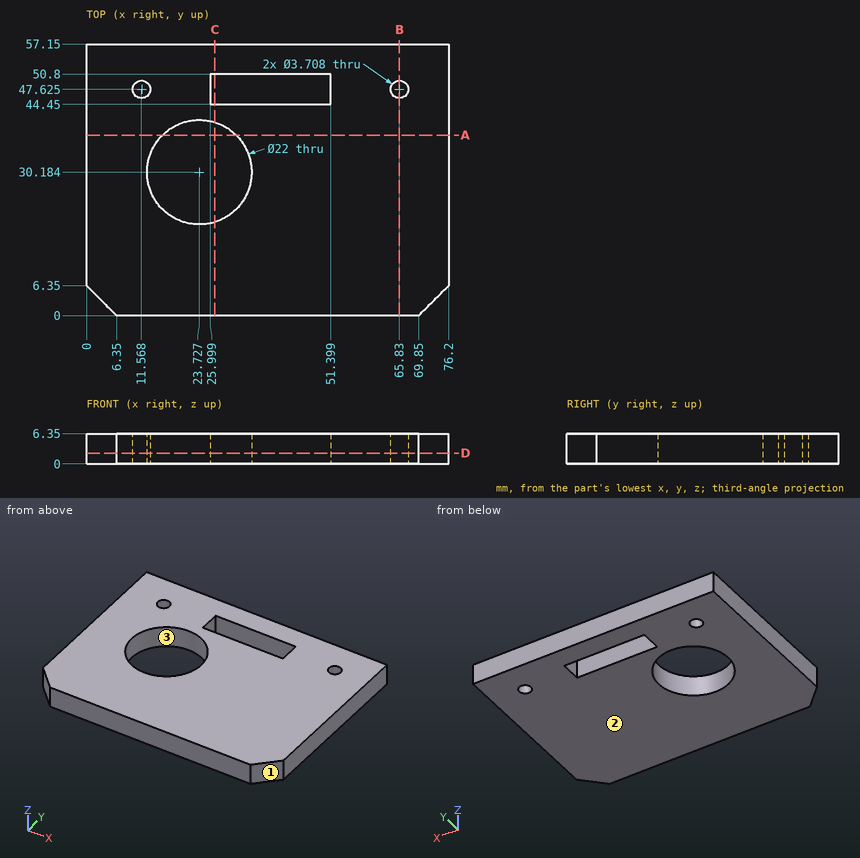
Drawing for the job (mm, zero at the part's lowest x, y, z). Coordinates: 2 decimals unless noted, no trailing zeros. Order: outer loops, then holes, each group sorted by start corner. A loop starts at its lowest first (then second) coordinate and runs counter-clockwise, first axis right, second up. Notation, with made-up numbers: (56, -13) - (63, -13) arc R18 ccw to (63, -7) - close; hole circle Ø10 at (-31.75, 66.25). An arc over 180 degrees is marked (long way). Use a Markdown table: item, result. Add a question column.
(1) Saw through at C-C (x = 27). Give the cut face in (y, z), then the cut area to 3 significant figures.
(2) Drill centre lines: line 1 along Y through (x, z) = (65.83, 4); line 2 along Y through (x, z) = (41.5, 4.25); line 3 along X through (y, z) = (46, 4) (1 decimal). Where is each one in solid material? Low to high. Write a range as [from, to].
(3) Saw through at B-B (x = 65.83). Give the cut face in (y, z), then the cut area to 3 significant figures.
(4) Pull direction X, two halves, no side cores. Call the marked faces 1, 2 and 3: +X half, -X half, draft (parallel to the pull), parting line (faces both ways), or undercut.
(5) Flat gauge pin, fed straight in: pin 1 (2 mm diameter, centred on x = 19.5, y = 10, fed in from -Z). Where does the tip first touch, or does it go through?
(6) Saw through at A-A (y = 38). Give the cut face in (x, z).
(7) Saw through at D-D (z = 2.25). Count the separate pieces of the cut face and the enclosed holes in it, then the cut area to 3 significant figures.
Solved:
| question | item | result |
|---|---|---|
| 1 | outline | (0, 0) - (19.68, 0) - (19.68, 6.35) - (0, 6.35) - close; (40.69, 0) - (44.45, 0) - (44.45, 6.35) - (40.69, 6.35) - close; (50.8, 0) - (57.15, 0) - (57.15, 6.35) - (50.8, 6.35) - close |
| 1 | area | 189 mm² |
| 2 | line 1 | y = [0, 45.77], [49.48, 57.15] |
| 2 | line 2 | y = [0, 44.45], [50.8, 57.15] |
| 2 | line 3 | x = [0, 10.7], [12.5, 26], [51.4, 64.9], [66.7, 76.2] |
| 3 | outline | (0, 0) - (45.77, 0) - (45.77, 6.35) - (0, 6.35) - close; (49.48, 0) - (57.15, 0) - (57.15, 6.35) - (49.48, 6.35) - close |
| 3 | area | 339 mm² |
| 4 | face 1 | +X half |
| 4 | face 2 | draft |
| 4 | face 3 | undercut |
| 5 | pin 1 | stops at z = 0 |
| 6 | outline | (0, 0) - (15.99, 0) - (15.99, 6.35) - (0, 6.35) - close; (31.47, 0) - (76.2, 0) - (76.2, 6.35) - (31.47, 6.35) - close |
| 7 | separate pieces | 1 |
| 7 | enclosed holes | 4 |
| 7 | area | 3,750 mm² |
